Source: CAD feature listing. Evaluate the final solid. Frame: model axes, mm. Give positions to 0.01 mm unless a question says otherwise; leave off trailing zeros. Write each loop counter-clockwise with the first axis right and the second up, starting at its lowest first coordinate (ties: lowest second). Pieces come first, ordered by that corner, then holes. Notation, with made-up numbers: (-3.75, 61) -> (23.25, 61) arc R14 ccw to (23.25, 86) -> close; hole circle Ø10 at (-28, 88). An arc over 180 degrees is marked (long way). Write item = value, one per line.
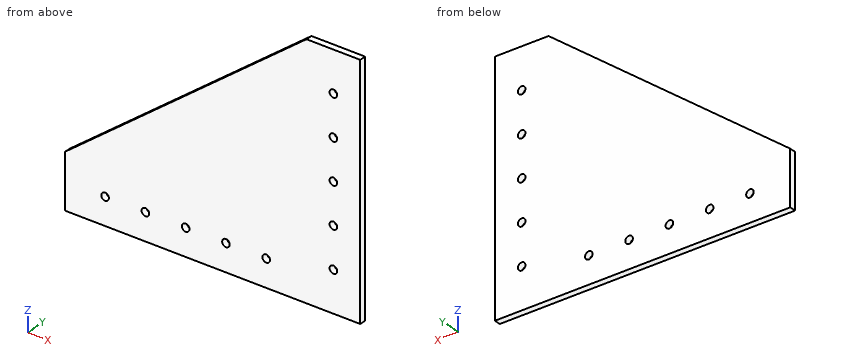
Autodesk Inventor part; units mm, degrees
ref_plane "YZ Plane" through (0, 0, 0) normal (1, 0, 0) x (0, 1, 0)
ref_plane "XZ Plane" through (0, 0, 0) normal (0, 1, 0) x (-1, 0, 0)
ref_plane "XY Plane" through (0, 0, 0) normal (0, 0, 1) x (1, 0, 0)
sketch "face_sketch" plane through (0, 0, 0) normal (0, 1, 0) x (-1, 0, 0)
  line L0 (0, 0) -> (0, -114.3)
  line L1 (139.7, -114.3) -> (139.7, -88.9)
  line L2 (139.7, -88.9) -> (25.4, 0)
  line L3 (25.4, 0) -> (0, 0)
  line L4 (25.4, 0) -> (25.4, -114.3) construction
  line L5 (0, -114.3) -> (25.4, -114.3)
  line L6 (25.4, -114.3) -> (139.7, -114.3)
  dimension "d0" = 114.3
  dimension "d2" = 25.4
  dimension "d3" = 25.4
  dimension "d5" = 114.3
extrude "Plate1" add sketch "face_sketch" along normal blind 3.048
sketch "Sketch4" plane through (0, 3.048, 0) normal (0, 1, 0) x (1, 0, 0)
  line L0 (-25.4, 0) -> (0, 0) construction
  line L1 (-12.7, 0) -> (-12.7, 19.05) construction
  line L2 (-12.7, 19.05) -> (-12.7, 38.1) construction
  line L3 (-12.7, 38.1) -> (-12.7, 57.15) construction
  line L4 (-12.7, 57.15) -> (-12.7, 76.2) construction
  line L5 (-12.7, 76.2) -> (-12.7, 95.25) construction
  line L6 (-12.7, 95.25) -> (-12.7, 114.3) construction
  line L7 (0, 114.3) -> (-139.7, 114.3) construction
  line L8 (-139.7, 114.3) -> (-139.7, 88.9) construction
  line L9 (-139.7, 101.6) -> (-120.65, 101.6) construction
  line L10 (-120.65, 101.6) -> (-101.6, 101.6) construction
  line L11 (-101.6, 101.6) -> (-82.55, 101.6) construction
  line L12 (-82.55, 101.6) -> (-63.5, 101.6) construction
  line L13 (-63.5, 101.6) -> (-44.45, 101.6) construction
  line L14 (-44.45, 101.6) -> (-25.4, 101.6) construction
  line L15 (-25.4, 0) -> (-25.4, 101.6) construction
hole "Hole1" at (-12.7, 3.048, -19.05) at (-12.7, 3.048, -38.1) at (-12.7, 3.048, -57.15) at (-12.7, 3.048, -76.2) at (-12.7, 3.048, -95.25) at (-120.65, 3.048, -101.6) at (-101.6, 3.048, -101.6) at (-82.55, 3.048, -101.6) at (-63.5, 3.048, -101.6) at (-44.45, 3.048, -101.6) direction (0, -1, 0) diameter 3.5719 depth 3.048 tip angle 118
equation "\"d6\" = rv_hole_diameter"
equation "\"d11\" = Thickness"
equation "\"d0\" = ncbt_rivet_row_length"
equation "\"d2\" = st_outer_diameter"
equation "\"d3\" = st_outer_diameter"
equation "\"d5\" = ncbt_rivet_row_length"
equation "\"BendRadius\" = Thickness"
equation "\"BendReliefWidth\" = Thickness"
equation "\"BendReliefDepth\" = 0.5 * Thickness"
equation "\"CornerReliefSize\" = 4 * Thickness"
equation "\"MinimumRemnant\" = 2 * Thickness"
equation "\"TransitionRadius\" = BendRadius"
equation "\"JacobiRadiusSize\" = BendRadius"
equation "\"GapSize\" = Thickness"
equation "\"bp_thickness\" = 3.048"
equation "\"bp_height\" = 25.4"
equation "\"bp_width\" = 25.4"
equation "\"bp_axle_height\" = 25.4"
equation "\"magic_axle_offset\" = 3.175"
equation "\"bp_tensioner_width\" = 6.35"
equation "\"bp_tensioner_height\" = 19.05"
equation "\"bp_tensioner_from_bottom\" = 50.8"
equation "\"bp_tensioner_from_side\" = 25.4"
equation "\"bp_tensioner_wood_mount_from_tensioner_top\" = 12.7"
equation "\"bp_tensioner_wood_mount_diameter\" = 6.35"
equation "\"gb_mh_seperation\" = 111.1504"
equation "\"gb_mh_diameter\" = 6.35"
equation "\"gb_axle_from_edge\" = 38.1"
equation "\"gb_width\" = 127"
equation "\"gb_bearing_diameter\" = 28.575"
equation "\"gb_to_bottom_of_side_assembly\" = 4.7752"
equation "\"rivet_row_length\" = 114.3"
equation "\"rv_hole_diameter\" = 3.57187"
equation "\"st_outer_diameter\" = 25.4"
equation "\"st_wall_thickness\" = 6.35"
equation "\"st_length\" = 939.8"
equation "\"st_gbmh_from_center\" = 0.5 * gb_mh_seperation"
equation "\"st_cutout_depth_right\" = 254"
equation "\"st_cutout_depth_left\" = 254"
equation "\"st_rivet_distance\" = 19.05"
equation "\"so_inner_diameter\" = 6.35"
equation "\"so_wall_thickness\" = 3.048"
equation "\"so_length\" = 25.4"
equation "\"twb_width\" = st_outer_diameter"
equation "\"twb_length\" = bp_tensioner_width + 2 * twb_margin_on_each_side"
equation "\"twb_height\" = 2 * bp_tensioner_wood_mount_diameter + bp_tensioner_height + 2 * bp_tensioner_wood_mount_from_tensioner_top + twb_margin_on_each_side"
equation "\"twb_margin_on_each_side\" = 6.35"
equation "\"twb_tensioner_from_edge\" = -0.5 * bp_tensioner_height + 0.5 * twb_height"
equation "\"tb_rivet_row_length\" = 127"
equation "\"ncbt_rivet_row_length\" = 114.3"
equation "\"d4\" = BendRadius"
properties part number "no_cutout_bracket_top(ncbt)"
1) Cut plane B-B (x = -101.6). Return the cut outline in (y, z), then the cut area to 3 significant figures.
Computed:
outline = (0, -114.3) -> (3.05, -114.3) -> (3.05, -103.39) -> (0, -103.39) -> close; (0, -99.81) -> (3.05, -99.81) -> (3.05, -59.27) -> (0, -59.27) -> close
area = 157 mm²
2) Material intervals for L1, parallel to X at y = 2.45, z = -101.6; L2, parallel to Z at x = -12.7, y = 1.8; L3, parallel to X at y = 1.1, z = -95.25, sorted ascending.
Computed:
L1 = -139.7 to -122.44, -118.86 to -103.39, -99.81 to -84.34, -80.76 to -65.29, -61.71 to -46.24, -42.66 to 0
L2 = -114.3 to -97.04, -93.46 to -77.99, -74.41 to -58.94, -55.36 to -39.89, -36.31 to -20.84, -17.26 to 0
L3 = -139.7 to -14.49, -10.91 to 0
3) Cut plane C-C (z = -38.1). Return the cut outline in (x, y).
Computed:
outline = (-74.39, 0) -> (-14.49, 0) -> (-14.49, 3.05) -> (-74.39, 3.05) -> close; (-10.91, 0) -> (0, 0) -> (0, 3.05) -> (-10.91, 3.05) -> close
4) Cut plane A-A (y = 0.55). State how many separate pieces and enclosed holes the cut face has, then the cut area to 3 significant figures.
Computed:
separate_pieces = 1
enclosed_holes = 10
area = 10,800 mm²
5) Cut plane D-D (x = -56). Return the cut outline in (y, z).
Computed:
outline = (0, -114.3) -> (3.05, -114.3) -> (3.05, -23.8) -> (0, -23.8) -> close
